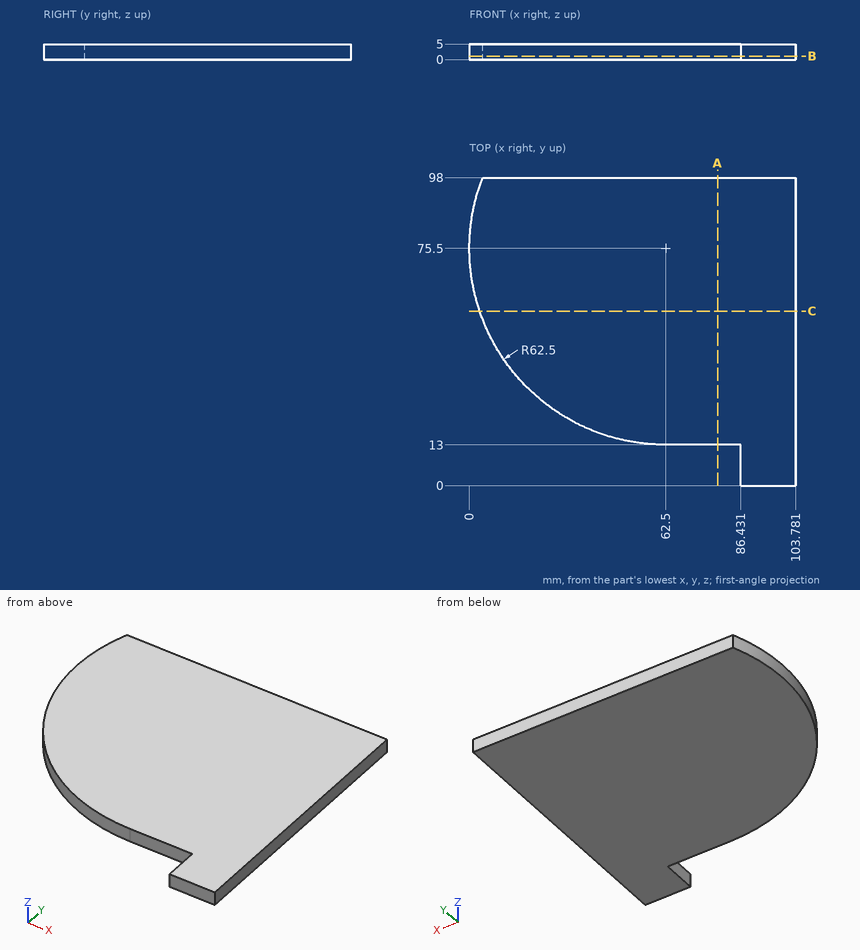
Job drawing, mm, ordinate dimensions from the low corner. One solid piece. Coordinates: 2 decimals unless noted, no trailing zeros. Write each loop counter-clockwise with the first axis right and the second up, starting at its lowest first coordinate (ties: lowest second). Pieces come first, ordered by that corner, then holes. Notation, with made-up numbers: (72, 20.5) - (108, 20.5) arc R15 ccw to (108, 40.5) - close; hole circle Ø10 at (26, 89.5). An arc over 180 degrees is marked (long way). Use a Markdown table: item, result. Add a question column.
Item 1: Band-saw the part on C-C, the plane y = 55.5. Give the cut face in (x, z).
Item 2: Band-saw the part on B-B, the plane z = 1.15. Give the cut face in (x, y).
Item 3: Flat gauge pins, fed straight in: pin 1 (3 mm diameter, centred on x = 82.5, z = 2, fed in from -Y); pin 2 (2 mm diameter, centred on y = 43, z = 3.5, fed in from -X). Where does each tip first touch, or does it go through?
Item 4: Band-saw the part on A-A, the plane x = 79. Give the cut face in (y, z).
Item 5: Drill centre lines: L1, parallel to Y at x = 67, z = 1; L2, parallel to X at y = 7, z = 4.5; L3, parallel to X at y = 68.5, z = 0.55. Where is each one in solid material? Low to high. Write a range as from..to.
Numbers:
| question | item | result |
|---|---|---|
| 1 | outline | (3.29, 0) - (103.78, 0) - (103.78, 5) - (3.29, 5) - close |
| 2 | outline | (4.19, 98) arc R62.5 ccw to (62.5, 13) - (86.43, 13) - (86.43, 0) - (103.78, 0) - (103.78, 98) - close |
| 3 | pin 1 | y = 13 |
| 3 | pin 2 | x = 8.52 |
| 4 | outline | (13, 0) - (98, 0) - (98, 5) - (13, 5) - close |
| 5 | L1 | 13..98 |
| 5 | L2 | 86.43..103.78 |
| 5 | L3 | 0.39..103.78 |
